The figure shows three views and two pictorial views of one solid part (mm, origin at its lowest corner). Answer the questions. Coordinates: 2 decimals unless noted, no trailing zeros. Loops run counter-clockwise (first coordinate to the right, second up) from the corner with the lowest first, then second, coordinate; pieces in that order, holes last. Notation, with made-up numbers: M 19,69.25 L 43,69.25 A33 ccw 43,107.25 Z; hole C 84,57.25 d6. An arc over 180 degrees is marked long. Write each question's results on one line, items separated by ' | '.
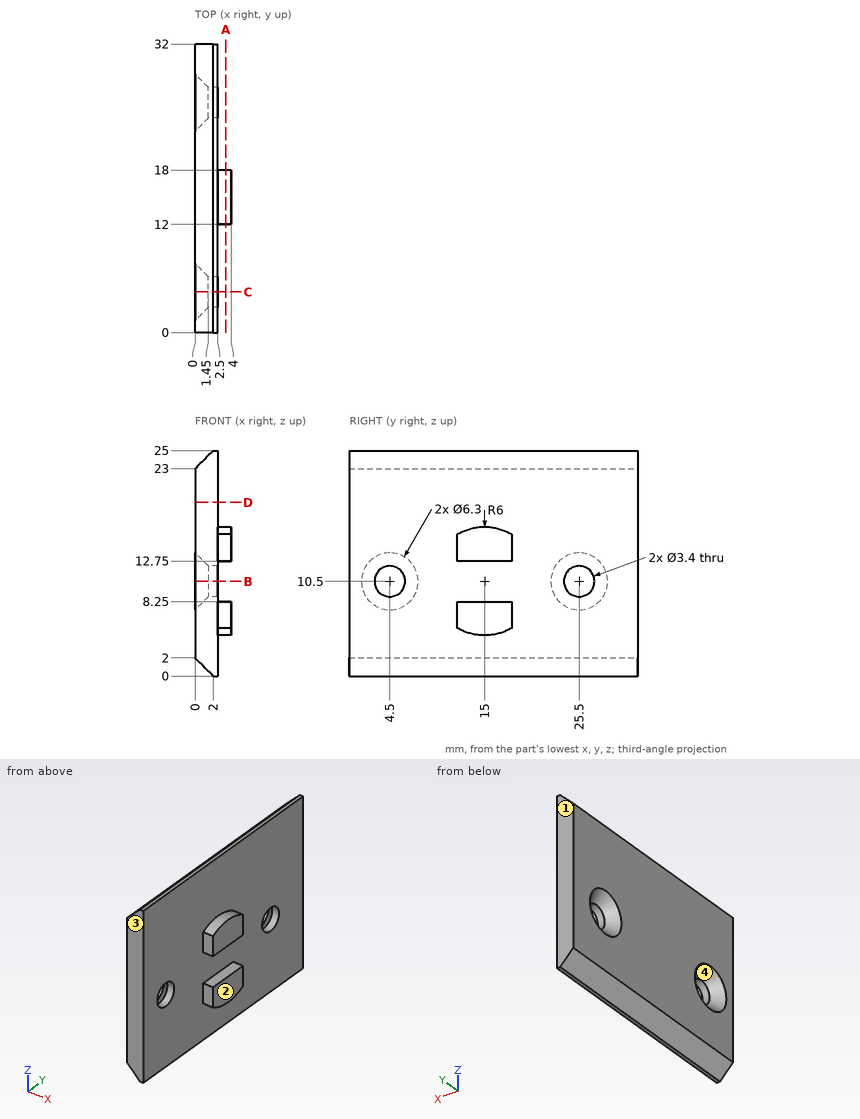
1) Find section D-D, the plane z = 19.25. Give the vertices of the cut face in (x, y).
Check result:
outline: M 0,0 L 2.5,0 L 2.5,32 L 0,32 Z
2) Find section B-B, the plane z = 10.5. Give the vertices of the cut face in (x, y), and give its area (3 significant figures).
Check result:
outline: M 0,0 L 2.5,0 L 2.5,2.8 L 1.45,2.8 L 0,1.35 Z; M 0,7.65 L 1.45,6.2 L 2.5,6.2 L 2.5,23.8 L 1.45,23.8 L 0,22.35 Z; M 0,28.65 L 1.45,27.2 L 2.5,27.2 L 2.5,32 L 0,32 Z | area: 58.8 mm^2
3) For a pull along Y with two mould halves and no side action, classify the marked faces 1, 2, 3 and 4 as released by +Y, released by -Y, zero draft, split by the parting line, or undercut.
Check result:
face 1: released by +Y | face 2: zero draft | face 3: released by -Y | face 4: undercut
4) Straight lines are drawn through the part: probe 1 along Y at (x, z) = (2.1, 10.5); probe 2 along Z at (x, y) = (2.1, 25.5); probe 3 along X at (y, z) = (30, 8.5). For each, find the intervals that lie inside material, in ascending order. Write a range as [from, to].
Check result:
probe 1: [0, 2.8], [6.2, 23.8], [27.2, 32] | probe 2: [0, 8.8], [12.2, 25] | probe 3: [0, 2.5]
5) Find section C-C, the plane y = 4.5. Give the vertices of the cut face in (x, z).
Check result:
outline: M 0,2 L 2,0 L 2.5,0 L 2.5,8.8 L 1.45,8.8 L 0,7.35 Z; M 0,13.65 L 1.45,12.2 L 2.5,12.2 L 2.5,25 L 2,25 L 0,23 Z
6) Find section A-A, the plane x = 3.4. Give the vertices of the cut face in (y, z), and give its area (3 significant figures).
Check result:
outline: M 12,5.3 A6 ccw 18,5.3 L 18,8.25 L 12,8.25 Z; M 12,12.75 L 18,12.75 L 18,15.7 A6 ccw 12,15.7 Z | area: 41.9 mm^2
7) Given pin 1 Ø12.5 at (y, z) = (10.5, 12.5) entering from +X; pin 2 Ø1.6 at (x, z) = (3.5, 14.5) entering from -Y; pin 3 Ø1.5 at (x, y) = (0.5, 21.5) entering from +Z; pin 4 Ø4.5 at (y, z) = (25.5, 10.5) entering from -X, each flat-ended and moving along its own axis, determine where each tip first touches the part or whether it passes through.
Check result:
pin 1: x = 4 | pin 2: y = 12 | pin 3: z = 24.25 | pin 4: x = 0.9
